Design review of the part built by this model. Coordinates are the model's own, in mm. A direction names the side the tool comes from. Give positions to 0.01 mm unless a question says otherwise; leave off trailing zeros. Loops run counter-clockwise (first coordinate to the right, second up) from the corner with the lowest first, then second, coordinate; pieces in that order, holes last. Notation, with made-up numbers: (-9.5, 13) - (43.5, 13) arc R34 cw to (43.5, 47) - close; hole circle Ø9 at (3, -16). An arc over 180 degrees is marked (long way). Put each result on its own line as item: value. Start each with the question number.
```python
from build123d import *

# Parameters (mm, degrees)
F1_DEPTH  = 19.05
F2_T      = -2.4
F4_DEPTH  = 14.11
F5_R      = 8.255
F5_R_2    = 6.35
F5_R_3    = 5.08
F6_DEPTH  = 30.2
F7_DEPTH  = 25.4
F8_DEPTH  = 34.5948
F9_R      = 8.255
F9_R_2    = 6.35
F9_R_3    = 5.08
F10_DEPTH = 30.2
F11_DEPTH = 25.4
F12_DEPTH = 36.9316
F13_R     = 8.255
F13_R_2   = 6.35
F13_R_3   = 5.08
F14_DEPTH = 30.2
F15_DEPTH = 25.4
F16_DEPTH = 31.242
F17_W     = 3.7311392443
F17_H     = 25.4
F17_W_2   = 25.4
F17_H_2   = 3.7311392443
F20_DEPTH = 2.54


with BuildPart() as f1:
    # F0 (on Top) → F1 (new body)
    with BuildSketch(Plane.XY):
        Polygon((-12.7, 25.4), (-38.1, 25.4), (-38.1, 0), (38.1, 0), (38.1, 25.4), (12.7, 25.4), (12.7, 50.8), (-12.7, 50.8), align=None)
    extrude(amount=F1_DEPTH)

    # F2
    f2_openings = [f1.faces().sort_by_distance(p)[0] for p in [
        (0, 19.05, 19.05),
    ]]
    offset(amount=F2_T, openings=f2_openings, kind=Kind.INTERSECTION)

    # F3 (on face) → F4 (join, through all)
    with BuildSketch(Plane.XY.offset(2.4)):
        Polygon((10.3, 48.4), (-10.3, 48.4), (-10.3, 23), (-35.7, 23), (-35.7, 2.4), (35.7, 2.4), (35.7, 23), (10.3, 23), align=None)
        Polygon((-33.3, 4.8), (-33.3, 20.6), (-7.9, 20.6), (-7.9, 46), (7.9, 46), (7.9, 20.6), (33.3, 20.6), (33.3, 4.8), align=None, mode=Mode.SUBTRACT)
    extrude(amount=F4_DEPTH)

    # F5 (on face) → F6 (join, through all)
    with BuildSketch(Plane(origin=(0, 50.8, 0), x_dir=(-1, 0, 0), z_dir=(0, 1, 0))):
        with Locations((0, 9.525)):
            Circle(F5_R)
        with Locations((0, 9.525)):
            Circle(F5_R_2, mode=Mode.SUBTRACT)
        with Locations((0, 9.525)):
            Circle(F5_R_2)
        with Locations((0, 9.525)):
            Circle(F5_R_3, mode=Mode.SUBTRACT)
        with Locations((0, 9.525)):
            Circle(F5_R_3)
    extrude(amount=-F6_DEPTH)

    # F5 (on face) → F7 (cut)
    with BuildSketch(Plane(origin=(0, 50.8, 0), x_dir=(-1, 0, 0), z_dir=(0, 1, 0))):
        with Locations((0, 9.525)):
            Circle(F5_R_2)
        with Locations((0, 9.525)):
            Circle(F5_R_3, mode=Mode.SUBTRACT)
        with Locations((0, 9.525)):
            Circle(F5_R_3)
    extrude(amount=-F7_DEPTH, mode=Mode.SUBTRACT)

    # F5 (on face) → F8 (cut)
    with BuildSketch(Plane(origin=(0, 50.8, 0), x_dir=(-1, 0, 0), z_dir=(0, 1, 0))):
        with Locations((0, 9.525)):
            Circle(F5_R_3)
    extrude(amount=-F8_DEPTH, mode=Mode.SUBTRACT)

    # F9 (on face) → F10 (join, through all)
    with BuildSketch(Plane.YZ.offset(38.1)):
        with Locations((12.7, 9.525)):
            Circle(F9_R)
        with Locations((12.7, 9.525)):
            Circle(F9_R_2, mode=Mode.SUBTRACT)
        with Locations((12.7, 9.525)):
            Circle(F9_R_2)
        with Locations((12.7, 9.525)):
            Circle(F9_R_3, mode=Mode.SUBTRACT)
        with Locations((12.7, 9.525)):
            Circle(F9_R_3)
    extrude(amount=-F10_DEPTH)

    # F9 (on face) → F11 (cut)
    with BuildSketch(Plane.YZ.offset(38.1)):
        with Locations((12.7, 9.525)):
            Circle(F9_R_2)
        with Locations((12.7, 9.525)):
            Circle(F9_R_3, mode=Mode.SUBTRACT)
    extrude(amount=-F11_DEPTH, mode=Mode.SUBTRACT)

    # F9 (on face) → F12 (cut)
    with BuildSketch(Plane.YZ.offset(38.1)):
        with Locations((12.7, 9.525)):
            Circle(F9_R_3)
    extrude(amount=-F12_DEPTH, mode=Mode.SUBTRACT)

    # F13 (on face) → F14 (join, through all)
    with BuildSketch(Plane(origin=(-38.1, 0, 0), x_dir=(0, -1, 0), z_dir=(-1, 0, 0))):
        with Locations((-12.7, 9.525)):
            Circle(F13_R)
        with Locations((-12.7, 9.525)):
            Circle(F13_R_2, mode=Mode.SUBTRACT)
        with Locations((-12.7, 9.525)):
            Circle(F13_R_2)
        with Locations((-12.7, 9.525)):
            Circle(F13_R_3, mode=Mode.SUBTRACT)
        with Locations((-12.7, 9.525)):
            Circle(F13_R_3)
    extrude(amount=-F14_DEPTH)

    # F13 (on face) → F15 (cut)
    with BuildSketch(Plane(origin=(-38.1, 0, 0), x_dir=(0, -1, 0), z_dir=(-1, 0, 0))):
        with Locations((-12.7, 9.525)):
            Circle(F13_R_2)
        with Locations((-12.7, 9.525)):
            Circle(F13_R_3, mode=Mode.SUBTRACT)
        with Locations((-12.7, 9.525)):
            Circle(F13_R_3)
    extrude(amount=-F15_DEPTH, mode=Mode.SUBTRACT)

    # F13 (on face) → F16 (cut)
    with BuildSketch(Plane(origin=(-38.1, 0, 0), x_dir=(0, -1, 0), z_dir=(-1, 0, 0))):
        with Locations((-12.7, 9.525)):
            Circle(F13_R_3)
    extrude(amount=-F16_DEPTH, mode=Mode.SUBTRACT)

    # F17 (on face) → F18 (join, up to the next surface of F1)
    with BuildSketch(Plane.XY.offset(2.4)):
        with Locations((-6.0344303778, 33.3)):
            Rectangle(F17_W, F17_H)
        with Locations((-20.6, 18.7344303778)):
            Rectangle(F17_W_2, F17_H_2)
        with Locations((6.0344303778, 33.3)):
            Rectangle(F17_W, F17_H)
        with Locations((-20.6, 6.6655696222)):
            Rectangle(F17_W_2, F17_H_2)
        with Locations((20.6, 18.7344303778)):
            Rectangle(F17_W_2, F17_H_2)
        with Locations((20.6, 6.6655696222)):
            Rectangle(F17_W_2, F17_H_2)
    extrude(until=Until.NEXT)

    # F19 (on face) → F20 (cut, through all)
    with BuildSketch(Plane.XY.offset(19.05)):
        Polygon((-10.3, 23), (-35.7, 23), (-35.7, 2.4), (35.7, 2.4), (35.7, 23), (10.3, 23), (10.3, 48.4), (-10.3, 48.4), align=None)
        Polygon((7.9, 46), (7.9, 20.6), (33.3, 20.6), (33.3, 17.0994090512), (33.3, 8.3005909488), (33.3, 4.8), (7.9, 4.8), (-7.9, 4.8), (-33.3, 4.8), (-33.3, 8.3005909488), (-33.3, 17.0994090512), (-33.3, 20.6), (-7.9, 20.6), (-7.9, 46), (-4.3994090512, 46), (4.3994090512, 46), align=None, mode=Mode.SUBTRACT)
        Polygon((-7.9, 20.6), (7.9, 20.6), (7.9, 46), (4.3994090512, 46), (-4.3994090512, 46), (-7.9, 46), align=None)
        Polygon((-7.9, 4.8), (-7.9, 20.6), (-33.3, 20.6), (-33.3, 17.0994090512), (-33.3, 8.3005909488), (-33.3, 4.8), align=None)
        Polygon((33.3, 20.6), (7.9, 20.6), (7.9, 4.8), (33.3, 4.8), (33.3, 8.3005909488), (33.3, 17.0994090512), align=None)
    extrude(amount=-F20_DEPTH, mode=Mode.SUBTRACT)


solid = f1.part
```
Item 1: Machinability: for faces 4 (the flat face through (-12.7, 38, 9)), 5 (the flat face through (-1, 20, 0)), 6 (the flat face through (-33.3, 6, 15)), 7 (the cylindrical face through (-25.58, 9.77, 3.89)), which of the approach directions +Z, -Z, +X, -X, +Y, -Y give a long, thin tool a straight path to every point of the face, cutting with its end or side? Answer none if there is none.
Item 2: For P1, Ø7.5, axis at x = 0, z = 9.525, coming from the +Y side; P2, Ø2.5, axis at y = 33.5, z = 15, coming from the +X side; P3, Ø1.4, axis at y = 35.5, z = 13.5, coming from the -X side, all flat-tipped, find the tip position at first contact; note any pin that passes through.
Item 3: Consider section A-A (y = 12.7). State the section outline as (x, z) points (3 decimals).
Item 4: Consider section B-B (z = 1.5). State the section outline as (x, y) points, plus the area to 3 significant figures.
Item 5: Consider section C-C (x = -29). State the section outline as (y, z) points (3 decimals).
Item 6: Consider section D-D (y = 30). State the section outline as (x, z) points (3 decimals), plus the area to 3 significant figures.
Item 7: Mouldability with a two-part tool opening along Z and no side actions: class faces 1 (the cylindrical face through (1.377, 38.278, 3.326)), 2 (the flat face through (-10.3, 36, 18)), 3 (the flat face through (0, 13, 2.4)) as pulls with the +Z half, pulls with the -Z half, needs draft (parallel to the pull), parting line crosses it, or undercut.
Item 8: For L1, parallel to Z at x = -20.5, y = 12.7 (3 decimals); L2, parallel to X at y = 3, z = 18.75; L3, parallel to X at y = 31.5, z = 16.75, list the stretches that pass through material, from the lowest coordinate up. Write a range as from..to.
Geometry says:
1. face 4: +Z, -Z, -X, +Y
1. face 5: -Z, +X, -X, +Y, -Y
1. face 6: +Z
1. face 7: -X
2. P1: stops at y = 4.8
2. P2: stops at x = 12.7
2. P3: stops at x = -12.7
3. outline: (-38.1, 0) - (38.1, 0) - (38.1, 3.175) - (12.7, 3.175) - (12.7, 4.445) - (7.9, 4.445) - (7.9, 2.4) - (-7.9, 2.4) - (-7.9, 4.445) - (-12.7, 4.445) - (-12.7, 3.175) - (-38.1, 3.175) - close; (-38.1, 15.875) - (-12.7, 15.875) - (-12.7, 14.605) - (-7.9, 14.605) - (-7.9, 16.51) - (-35.7, 16.51) - (-35.7, 19.05) - (-38.1, 19.05) - close; (7.9, 14.605) - (12.7, 14.605) - (12.7, 15.875) - (38.1, 15.875) - (38.1, 19.05) - (35.7, 19.05) - (35.7, 16.51) - (7.9, 16.51) - close
4. outline: (-38.1, 0) - (38.1, 0) - (38.1, 25.4) - (12.7, 25.4) - (12.7, 50.8) - (-12.7, 50.8) - (-12.7, 25.4) - (-38.1, 25.4) - close
4. area: 2,580 mm2
5. outline: (0, 0) - (25.4, 0) - (25.4, 19.05) - (23, 19.05) - (23, 16.51) - (20.6, 16.51) - (20.6, 11.92) arc R8.255 ccw to (17.099, 16.51) - (8.301, 16.51) arc R8.255 ccw to (4.8, 11.92) - (4.8, 16.51) - (2.4, 16.51) - (2.4, 19.05) - (0, 19.05) - close; hole circle Ø12.7 at (12.7, 9.525)
6. outline: (-12.7, 0) - (12.7, 0) - (12.7, 19.05) - (10.3, 19.05) - (10.3, 16.51) - (7.9, 16.51) - (7.9, 11.92) arc R8.255 ccw to (4.399, 16.51) - (-4.399, 16.51) arc R8.255 ccw to (-7.9, 11.92) - (-7.9, 16.51) - (-10.3, 16.51) - (-10.3, 19.05) - (-12.7, 19.05) - close; hole circle Ø12.7 at (0, 9.525)
6. area: 293 mm2
7. face 1: undercut
7. face 2: needs draft
7. face 3: pulls with the +Z half
8. L1: z = 0..3.175, 15.875..16.51
8. L2: x = -38.1..-35.7, 35.7..38.1
8. L3: x = -12.7..-10.3, 10.3..12.7
